The listing builds one solid part. Answer for the finished solid, in the listing's coordinates (mm). Coordinates: 2 decimals unless noted, no trailing zeros. Order: outer loops, then holes, each group sorted by start corner. A loop starts at its lowest first (then second) coordinate and runs counter-clockwise, first axis right, second up. Notation, with made-up numbers: M 87.5,45.25 L 141.5,45.25 A25 cw 141.5,67.25 Z; hole C 41.25,-29 d6. An arc over 180 degrees is marked long. One line per item, written item: value. Start each with the question number.
Q1. Straight lines are drawn through the part: line 1 along X through (y, z) = (0, 3.35); line 2 along X through (y, z) = (-1.25, 2.7). For each, find the intervals that lie inside material, in ascending order. Write a range as [from, to].
Q2. The part is cut by section B-B on z = 1.2. Give the vertices of the cut face in (x, y), then the cut area to 3 significant figures.
Q3. The part is cut by section A-A on x = 0. Give the vertices of the cut face in (y, z).
Q4. Determine the mould class of faces 1 (the cylindrical face through (4.699, 4.715, 2.535)), 2 (the cylindrical face through (-0.631, -2.003, 2.528)), 3 (the cylindrical face through (-4.715, 4.699, 2.535)), 4 (the flat face through (2, 2, 0)) for opening direction X: pulls with the +X half, pulls with the -X half, needs draft (parallel to the pull), parting line crosses it, or undercut.
```python
from build123d import *

# Parameters (mm, degrees)
SKETCH_1_W      = 10
SKETCH_1_H      = 10
EXTRUDE_1_DEPTH = 5
FILLET_1_R      = 1


with BuildPart() as part:
    # Эскиз1 → Бобышка-Вытянуть1 (new body)
    with BuildSketch(Plane.XY):
        Rectangle(SKETCH_1_W, SKETCH_1_H)
    extrude(amount=EXTRUDE_1_DEPTH)

    # Эскиз3 → Отверстие обработанное метчиком M51 (revolve, cut)
    with BuildSketch(Plane(origin=(0, 0, 5), x_dir=(0, -1, 0), z_dir=(1, 0, 0))):
        Polygon((0, 0), (0, 5), (2.6, 5), (2.1, 4.5), (2.1, 0.5), (2.6, 0), align=None)
    revolve(axis=Axis((0, 0, 11.35), (0, 0, -1)), mode=Mode.SUBTRACT)

    # Скругление1
    fillet_1_edges = [part.edges().sort_by_distance(p)[0] for p in [
        (5, -5, 2.5),
        (-5, -5, 2.5),
        (-5, 5, 2.5),
        (5, 5, 2.5),
    ]]
    fillet(fillet_1_edges, radius=FILLET_1_R)


solid = part.part
```
Output:
1. line 1: x = [-5, -2.1], [2.1, 5]
1. line 2: x = [-5, -1.69], [1.69, 5]
2. outline: M -5,-4 A1 ccw -4,-5 L 4,-5 A1 ccw 5,-4 L 5,4 A1 ccw 4,5 L -4,5 A1 ccw -5,4 Z; hole C 0,0 d4.2
2. area: 85.3 mm^2
3. outline: M -5,0 L -2.6,0 L -2.1,0.5 L -2.1,4.5 L -2.6,5 L -5,5 Z; M 2.1,0.5 L 2.6,0 L 5,0 L 5,5 L 2.6,5 L 2.1,4.5 Z
4. face 1: pulls with the +X half
4. face 2: undercut
4. face 3: pulls with the -X half
4. face 4: needs draft
